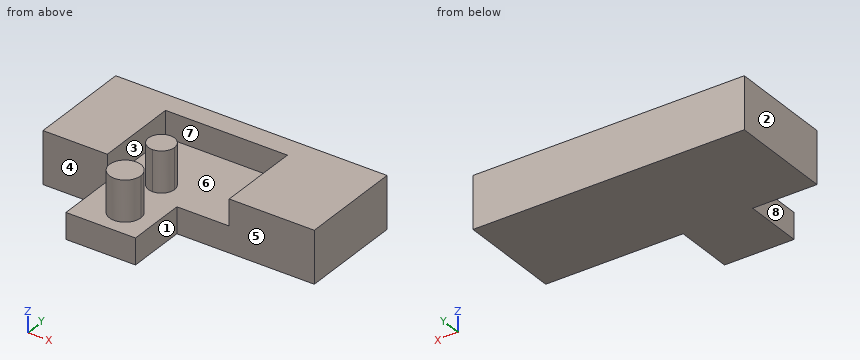
from build123d import *

# Parameters (mm, degrees)
F1_DEPTH = 25
F3_DEPTH = 25
F5_DEPTH = 39


with BuildPart() as f1:
    # F0 (on Top) → F1 (new body)
    with BuildSketch(Plane.XY):
        Polygon((-120.090559, 100), (-120.090559, 0), (-58.279246, 0), (-58.279246, 80), (58.720754, 80), (58.720754, 0), (140.4, 0), (140.4, 100), align=None)
    extrude(amount=F1_DEPTH)

    # F2 (on face) → F3 (join)
    with BuildSketch(Plane(origin=(0, 0, 0), x_dir=(1, 0, 0), z_dir=(0, 0, -1))):
        Polygon((-58.279246, 0), (-120.090559, 0), (-120.090559, -100), (140.4, -100), (140.4, 0), (8.472341, 0), (8.472341, 56.960292), (-58.279246, 56.960292), align=None)
    extrude(amount=F3_DEPTH)

    # F4 (on face) → F5 (join)
    with BuildSketch(Plane.XY):
        with BuildLine():
            ThreePointArc((-20.279246, 7.5), (-11.440411, 11.161165), (-7.779246, 20))
            ThreePointArc((-7.779246, 20), (-29.118081, 28.838835), (-20.279246, 7.5))
        make_face()
        with BuildLine():
            ThreePointArc((-5.279246, -30), (-9.672644, -19.393398), (-20.279246, -15))
            ThreePointArc((-20.279246, -15), (-30.885847, -40.606602), (-5.279246, -30))
        make_face()
    extrude(amount=F5_DEPTH)


solid = f1.part
Input: part model. Units: mm. Frame: model coordinates. Face numbers are marked on the shaded views. A direction names the side the tool comes from. Round coordinates to 2 decimals unless told otherwise and drop trailing zeros. Order: outer loops, then holes, each group sorted by start corner. A loop starts at its lowest first (then second) coordinate and runs counter-clockwise, first axis right, second up. Notation, with made-up numbers: (50.5, 31.25) - (93.5, 31.25) arc R35 cw to (93.5, 68.25) - close; hole circle Ø4 at (-2, 29.5). An arc over 180 degrees is marked (long way). Answer as a JSON object with one key per item and string values. Group by question number.
(1) Cut plane C-C (x = 2). Return loops of the section in (y, z), then the cut area to 3 significant figures.
(2) Reachability of the marked faces 1, 2, 3 and 4 from +Z, -Z, +X, -X, +Y, -Y: full face, straight path, thin tool, end or side. Return the list, or none.
(3) Material intervals for probe 1 along X at (y, z) = (19.5, 19); probe 2 along X at (y, z) = (16.5, 15); probe 3 along X at (y, z) = (75, 9.5), sorted ascending. Write a range as from..to.
(4) Draft query along Y for the marked faces 5, 6, 7 and 8. Return one class per face: released by +Y, released by -Y, zero draft, split by the parting line, or undercut.
(5) Cut plane B-B (z = 29.5). Return loops of the section in (x, y), then the cut area to 3 significant figures.
(6) Cut plane A-A (y = 66). Return loops of the section in (x, z).
(7) Pin query (flat end, axial travel): P1, Ø12.5, axis at y = -14.5, z = -15, coming from the +X side; P2, Ø4, axis at y = -3, z = -16, coming from the -X side; P3, Ø8, axis at x = 4.5, z = 14.5, coming from the -Y side. Return the tip coordinate at first contact, or that it passes through.
(8) Cut plane D-D (y = 25.5). Return loops of the section in (x, z).
Here are the results:
{
 "1": {"outline": "(-56.96, -25) - (100, -25) - (100, 25) - (80, 25) - (80, 0) - (-56.96, 0) - close", "area": "4,420 mm^2"},
 "2": {"face 1": "+Z, -Z, +X, -Y", "face 2": "+Z, -Z, -X, +Y, -Y", "face 3": "+Z, -Y", "face 4": "+Z, -Z, -X, -Y"},
 "3": {"probe 1": "x = -120.09..-58.28, -32.77..-7.79, 58.72..140.4", "probe 2": "x = -120.09..-58.28, -32.28..-8.28, 58.72..140.4", "probe 3": "x = -120.09..-58.28, 58.72..140.4"},
 "4": {"face 5": "released by -Y", "face 6": "undercut", "face 7": "undercut", "face 8": "zero draft"},
 "5": {"outline": "circle Ø30 at (-20.28, -30); circle Ø25 at (-20.28, 20)", "area": "1,200 mm^2"},
 "6": {"outline": "(-120.09, -25) - (140.4, -25) - (140.4, 25) - (58.72, 25) - (58.72, 0) - (-58.28, 0) - (-58.28, 25) - (-120.09, 25) - close"},
 "7": {"P1": "stops at x = 8.47", "P2": "stops at x = -58.28", "P3": "stops at y = 80"},
 "8": {"outline": "(-120.09, -25) - (140.4, -25) - (140.4, 25) - (58.72, 25) - (58.72, 0) - (-9.05, 0) - (-9.05, 39) - (-31.5, 39) - (-31.5, 0) - (-58.28, 0) - (-58.28, 25) - (-120.09, 25) - close"}
}
